Geometry: final body of the model. Coordinates: model frame, mm. Face numbers are marked on the shaded views. A direction names the side the tool comes from. Coordinates: 2 decimals unless noted, no trailing zeros. Loops run counter-clockwise (first coordinate to the right, second up) from the corner with the lowest first, then second, coordinate; pieces in that order, holes last. Notation, with made-up numbers: (-28, 8.25) -> (7, 8.25) arc R12 cw to (7, 29.25) -> close; hole circle Ø10 at (81.25, 84.5). An arc over 180 degrees is marked (long way). One line per item, written item: value. Start each with the question number.
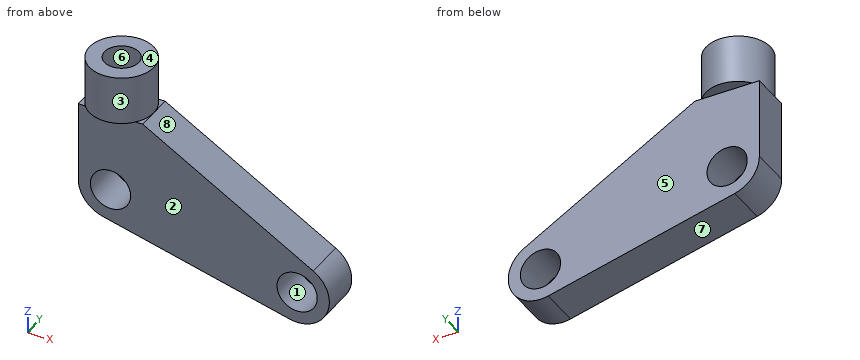
Autodesk Inventor part; units mm, degrees
ref_plane "YZ Plane" through (0, 0, 0) normal (1, 0, 0) x (0, 1, 0)
ref_plane "XZ Plane" through (0, 0, 0) normal (0, 1, 0) x (-1, 0, 0)
ref_plane "XY Plane" through (0, 0, 0) normal (0, 0, 1) x (1, 0, 0)
sketch "Sketch1" plane through (0, 0, 0) normal (0, 1, 0) x (-1, 0, 0)
  circle A0 centre (0, 0) radius 3.175
  arc A1 (1.2165, -4.9322) -> (5.08, 0) centre (0, 0) ccw
  line L0 (5.08, 0) -> (5.08, 12.7)
  line L1 (0, 0) -> (-5.08, 0) construction
  line L2 (-5.08, 0) -> (-29.4214, -7.2565) construction
  line L3 (-5.08, 0) -> (20.32, 0) construction
  arc A2 (-31.9659, -2.8597) -> (-28.2049, -12.1887) centre (-29.4214, -7.2565) ccw
  circle A3 centre (-29.4214, -7.2565) radius 3.175
  line L4 (5.08, 12.7) -> (-5.08, 12.7)
  line L5 (-5.08, 12.7) -> (-31.9659, -2.8597)
  line L6 (1.2165, -4.9322) -> (-28.2049, -12.1887)
  dimension "d0" = 6.35
  dimension "d1" = 10.16
  dimension "d2" = 12.7
  dimension "d3" = 25.4
  dimension "d4" = 163.4
  dimension "d5" = 10.16
  dimension "d6" = 6.35
  dimension "d7" = 10.16
extrude "Extrusion1" add sketch "Sketch1" along normal blind 6.35
sketch "Sketch2" plane through (-5.08, 0, 12.7) normal (0, 0, 1) x (1, 0, 0)
  line L0 (5.08, 0) -> (5.08, 6.35) construction
  line L1 (0, 6.35) -> (10.16, 6.35) construction
  circle A0 centre (5.08, 3.175) radius 5.08
  dimension "d10" = 10.16
extrude "Extrusion2" add sketch "Sketch2" along normal blind 7.62
sketch "Sketch4" plane through (0, 3.175, 20.32) normal (0, 0, 1) x (1, 0, 0)
  point P0 (0, -3.175)
  point P1 (0, 0)
hole "Hole1" at (0, 3.175, 20.32) direction (0, 0, -1) diameter 5.3975 depth 10.16 tip angle 118
properties part number "StteringArm"
1. Section B-B on z = -6. Return the cut outline in (x, y), plus the area to 3 significant figures.
2. Section A-A on x = 30.5. Return the cut outline in (y, z), plus the area to 3 significant figures.
3. Section D-D on y = 7.25. Return the cut outline in (x, z), plus the area to 3 significant figures.
4. Section C-C on z = 13.5. Return the cut outline in (x, y) (1 decimal).
5. Draft query along X for the marked faces 6, 7 and 8. Return one class per face: released by +X, released by -X, zero draft, split by the parting line, or undercut.
6. Pin query (flat end, axial travel): pin 1 Ø2 at (x, y) = (-1.5, 7.5) entering from -Z; pin 2 Ø4 at (x, y) = (9, 5.5) entering from +Z; pin 3 Ø3 at (x, y) = (0, 3.175) entering from +Z. Return the tip coordinate at first contact, or that it passes through.
7. Line query: L1, parallel to Y at x = 16.5, z = -5; L2, parallel to X at y = 1, z = 16; L3, parallel to Z at x = 27, y = 2. Output: solid intervals per line, ascending. Write a range as [from, to].
8. Set-up query: the marked faces 1, 2, 3, 4 and 5. Return all of +Z, -Z, +X, -X, +Y, -Y with unobstructed straight access to the full face (end or side cutting, diameter ignored); none if empty.
Checks:
1. outline: (3.11, 0) -> (26.51, 0) -> (26.51, 6.35) -> (3.11, 6.35) -> close; (32.34, 0) -> (34.34, 0) -> (34.34, 6.35) -> (32.34, 6.35) -> close
1. area: 161 mm²
2. outline: (0, -12.22) -> (6.35, -12.22) -> (6.35, -10.24) -> (0, -10.24) -> close; (0, -4.27) -> (6.35, -4.27) -> (6.35, -2.01) -> (0, -2.01) -> close
2. area: 26.9 mm²
3. outline: (-3.03, 12.7) -> (3.03, 12.7) -> (3.03, 20.32) -> (-3.03, 20.32) -> close
3. area: 46.2 mm²
4. outline: circle Ø10.2 at (0, 3.2); hole circle Ø5.4 at (0, 3.2)
5. face 6: undercut
5. face 7: released by -X
5. face 8: released by +X
6. pin 1: z = 12.7
6. pin 2: z = 11.59
6. pin 3: z = 9.44
7. L1: [0, 6.35]
7. L2: [-4.59, -1.6], [1.6, 4.59]
7. L3: [-11.89, -9.31], [-5.2, 0.01]
8. face 1: +Y, -Y
8. face 2: -Z, +X, -X, -Y
8. face 3: +Z
8. face 4: +Z, +X, -X, +Y, -Y
8. face 5: -Z, +X, -X, +Y
